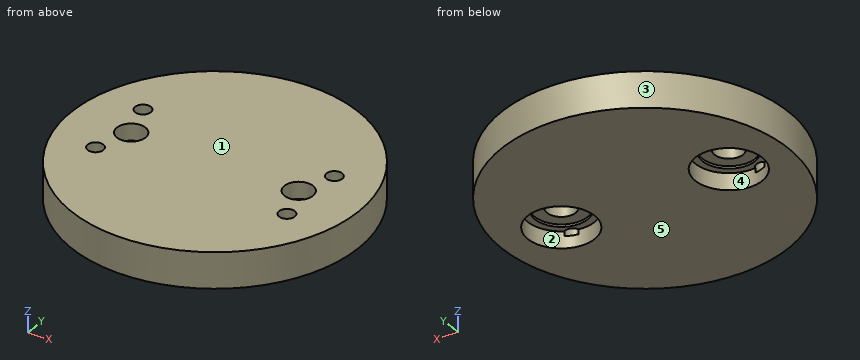
from build123d import *

# Parameters (mm, degrees)
SKETCH_1_R          = 60
EXTRUDE_1_DEPTH     = 15
SKETCH_2_R          = 6
CUT_EXTRUDE_1_DEPTH = 87.168439698
SKETCH_3_R          = 11
CUT_EXTRUDE_2_DEPTH = 8
SKETCH_5_R          = 3.3
CUT_EXTRUDE_4_DEPTH = 10
SKETCH_6_R          = 14
CUT_EXTRUDE_5_DEPTH = 7


with BuildPart() as part:
    # 草图1 → 凸台-拉伸1 (new body)
    with BuildSketch(Plane.XY):
        Circle(SKETCH_1_R)
    extrude(amount=EXTRUDE_1_DEPTH)

    # 草图2 → 切除-拉伸1 (cut, through all)
    with BuildSketch(Plane(origin=(0, 0, 0), x_dir=(-1, 0, 0), z_dir=(0, 0, -1))):
        with Locations((-35, 0)):
            Circle(SKETCH_2_R)
        with Locations((35, 0)):
            Circle(SKETCH_2_R)
    extrude(amount=-CUT_EXTRUDE_1_DEPTH, mode=Mode.SUBTRACT)

    # 草图3 → 切除-拉伸2 (cut)
    with BuildSketch(Plane(origin=(0, 0, 0), x_dir=(-1, 0, 0), z_dir=(0, 0, -1))):
        with Locations((35, 0)):
            Circle(SKETCH_3_R)
        with Locations((-35, 0)):
            Circle(SKETCH_3_R)
    extrude(amount=-CUT_EXTRUDE_2_DEPTH, mode=Mode.SUBTRACT)

    # 草图5 → 切除-拉伸4 (cut)
    with BuildSketch(Plane.XY.offset(15)):
        with Locations((40, 15)):
            Circle(SKETCH_5_R)
        with Locations((40, -15)):
            Circle(SKETCH_5_R)
        with Locations((-40, -15)):
            Circle(SKETCH_5_R)
        with Locations((-40, 15)):
            Circle(SKETCH_5_R)
    extrude(amount=-CUT_EXTRUDE_4_DEPTH, mode=Mode.SUBTRACT)

    # 草图6 → 切除-拉伸5 (cut)
    with BuildSketch(Plane(origin=(0, 0, 0), x_dir=(-1, 0, 0), z_dir=(0, 0, -1))):
        with Locations((35, 0)):
            Circle(SKETCH_6_R)
        with Locations((-35, 0)):
            Circle(SKETCH_6_R)
    extrude(amount=-CUT_EXTRUDE_5_DEPTH, mode=Mode.SUBTRACT)


solid = part.part
CAD build for the part. Positions are in the model's coordinates, mm. Face numbers are marked on the shaded views. A direction names the side the tool comes from. Round coordinates to 2 decimals unless told otherwise and drop trailing zeros. Write each loop counter-clockwise with the first axis right and the second up, starting at its lowest first coordinate (ties: lowest second). Pieces come first, ordered by that corner, then holes. Notation, with made-up numbers: (83, 20.25) -> (112, 20.25) arc R25 cw to (112, 41.25) -> close; hole circle Ø6 at (61, 7.5). An arc over 180 degrees is marked (long way). Answer as a JSON object with one key per item and string values.
(1) Band-saw the part on A-A, the plane y = 0. List the corners of the cut face in (x, z), then the cut area to 3 significant figures.
Reported:
{"outline": "(-60, 0) -> (-49, 0) -> (-49, 7) -> (-46, 7) -> (-46, 8) -> (-41, 8) -> (-41, 15) -> (-60, 15) -> close; (-29, 8) -> (-24, 8) -> (-24, 7) -> (-21, 7) -> (-21, 0) -> (21, 0) -> (21, 7) -> (24, 7) -> (24, 8) -> (29, 8) -> (29, 15) -> (-29, 15) -> close; (41, 8) -> (46, 8) -> (46, 7) -> (49, 7) -> (49, 0) -> (60, 0) -> (60, 15) -> (41, 15) -> close", "area": "1,200 mm^2"}
(2) Two-plate mould, pull along X, no slides. Class the marked faces 3, 4 and 5: +X half, -X half, draft (parallel to the pull), parting line (faces both ways), or undercut.
Reported:
{"face 3": "parting line", "face 4": "undercut", "face 5": "draft"}
(3) Pin check, flat tips, straight feed: P1, Ø6, axis at y = -7, z = 7, coming from the +X side; P2, Ø4, axis at x = 40, y = -15, coming from the +Z side; P3, Ø8.5, axis at x = -31, y = 6, coming from the -Z side; P4, Ø11, axis at x = 35, y = 0, coming from the -Z side. Stop position of each tip, or through.
Reported:
{"P1": "stops at x = 59.87", "P2": "stops at z = 5", "P3": "stops at z = 7", "P4": "passes through"}
(4) Which spindle directions (+Z, -Z, +X, -X, +Y, -Y) get a long thin tool onto all of the face, cutting with end or side? Do the marked faces 1 and 2. Say none if no direction does.
Reported:
{"face 1": "+Z, +X, -X, +Y, -Y", "face 2": "-Z"}
(5) Band-saw the part on D-D, the plane y = -22. List the corners of the cut face in (x, z), then the cut area to 3 significant figures.
Reported:
{"outline": "(-55.82, 0) -> (55.82, 0) -> (55.82, 15) -> (-55.82, 15) -> close", "area": "1,670 mm^2"}
(6) Band-saw the part on C-C, the plane x = 11. List the corners of the cut face in (y, z).
Reported:
{"outline": "(-58.98, 0) -> (58.98, 0) -> (58.98, 15) -> (-58.98, 15) -> close"}
(7) Probe probe 1 along X at (y, z) = (15, 11.5); probe 2 along Y at (x, z) = (40.5, 13.5); probe 3 along Y at (x, z) = (40, 8.25). List the from-to ranges inside material, lowest first. Write a range as [from, to].
Reported:
{"probe 1": "x = [-58.09, -43.3], [-36.7, 36.7], [43.3, 58.09]", "probe 2": "y = [-44.27, -18.26], [-11.74, -2.4], [2.4, 11.74], [18.26, 44.27]", "probe 3": "y = [-44.72, -18.3], [-11.7, -3.32], [3.32, 11.7], [18.3, 44.72]"}
(8) Band-saw the part on B-B, the plane z = 3.5. List the corners of the cut face in (x, y).
Reported:
{"outline": "circle Ø120 at (0, 0); hole circle Ø28 at (-35, 0); hole circle Ø28 at (35, 0)"}
